CAD build for the part. Positions are in the model's coordinates, mm. A direction names the side the tool comes from. Round coordinates to 2 decimals unless told otherwise and drop trailing zeros. Order: outer loops, then holes, each group sorted by start corner. A loop starts at its lowest first (then second) coordinate and runs counter-clockwise, first axis right, second up. Notation, with made-up numbers: (39, -34) -> (92, -34) arc R21 cw to (92, -23) -> close; hole circle Ø8 at (-37, 1). An arc over 180 degrees is marked (long way). Return JSON: item names as keys, results as strings. Group by question number.
Q1. Which spindle directions (+Z, -Z, +X, -X, +Y, -Y) get a long thin tool onto all of the face, cutting with end or side? Do faces 4 (the flat face through (-27, 64, 5)), 5 (the flat face through (19, 240, -4)). Say none if no direction does.
Q2. Cut at B-B (x = 0). Write the cut outline in (y, z).
Q3. Cut at A-A (z = 0). Write the cut outline in (x, y).
Q4. Cut at D-D (x = 31). Count the separate pieces of the cut face and the enclosed holes in it, then the cut area to 3 significant figures.
Q5. Mould opens along Z. For faces 1 (the flat face through (27, 156, 0)), 2 (the cylindrical face through (-34.168, 118.46, -7.587)), 3 (the flat face through (19, 0, -4)) say: +Z half, -Z half, draft (parallel to the pull), parting line (faces both ways), or undercut.
Q6. Cut at C-C (y = 54). Write the cut outline in (x, z).
Q7. Probe line 1 along Y through (x, z) = (-29, 0.5); line 2 along Z through (x, y) = (-24.5, 75.5) (3 decimals); line 3 along Y through (x, z) = (4, 25.5). List the from-to ranges inside material, lowest first.
Q8. Flat gauge pins, fed straight in: pin 1 (8 mm diameter, centred on x = -29.5, z = 0.5, fed in from +Y); pin 2 (5 mm diameter, centred on x = -28.5, y = 180.5, fed in from +Z); pin 3 (3 mm diameter, centred on x = 8, y = 134, fed in from -Z). Where does each tip first touch, or does it go through?
from build123d import *

# Parameters (mm, degrees)
SKETCH3_R               = 35
SKETCH3_R_2             = 19
BOSS_EXTRUDE2_DEPTH     = 240
CUT_EXTRUDE2_DEPTH      = 246.051015097
CUT_EXTRUDE2_DEPTH_BACK = 246.051015097
SKETCH5_W               = 10
SKETCH5_H               = 40
CUT_EXTRUDE3_DEPTH      = 246.051015097
CUT_EXTRUDE3_DEPTH_BACK = 246.051015097
SKETCH6_W               = 10
SKETCH6_H               = 40
FILLET2_R               = 10
FILLET3_R               = 10


with BuildPart() as part:
    # Sketch3 → Boss-Extrude2 (new body)
    with BuildSketch(Plane(origin=(0, 0, 0), x_dir=(1, 0, 0), z_dir=(0, 1, 0))):
        with Locations(Location((0, 0, 0), (0, 0, 270))):
            Circle(SKETCH3_R)
        with Locations(Location((0, 0, 0), (0, 0, 270))):
            Circle(SKETCH3_R_2, mode=Mode.SUBTRACT)
    extrude(amount=BOSS_EXTRUDE2_DEPTH)

    # Sketch5 → Cut-Extrude2 (cut, two sides: drawn at the far end of the back side and taken through both)
    with BuildSketch(Plane(origin=(0, 0, 0), x_dir=(0, 0, -1), z_dir=(1, 0, 0)).offset(-CUT_EXTRUDE2_DEPTH_BACK)):
        with Locations((0, 176)):
            Rectangle(SKETCH5_W, SKETCH5_H)
    extrude(amount=CUT_EXTRUDE2_DEPTH + CUT_EXTRUDE2_DEPTH_BACK, mode=Mode.SUBTRACT)

    # Sketch6 → Cut-Extrude3 (cut, two sides: drawn at the far end of the back side and taken through both)
    with BuildSketch(Plane(origin=(0, 0, 0), x_dir=(0, 0, -1), z_dir=(1, 0, 0)).offset(-CUT_EXTRUDE3_DEPTH_BACK)):
        with Locations((0, 64)):
            Rectangle(SKETCH6_W, SKETCH6_H)
    extrude(amount=CUT_EXTRUDE3_DEPTH + CUT_EXTRUDE3_DEPTH_BACK, mode=Mode.SUBTRACT)

    # Fillet2
    fillet2_edges = [part.edges().sort_by_distance(p)[0] for p in [
        (0, 240, -35),
    ]]
    fillet(fillet2_edges, radius=FILLET2_R)

    # Fillet3
    fillet3_edges = [part.edges().sort_by_distance(p)[0] for p in [
        (0, 0, -35),
    ]]
    fillet(fillet3_edges, radius=FILLET3_R)


solid = part.part
Solution:
{
 "1": {"face 4": "+X, -X", "face 5": "+Z, -Z, +X, -X, +Y"},
 "2": {"outline": "(0, -25) arc R10 ccw to (10, -35) -> (230, -35) arc R10 ccw to (240, -25) -> (240, -19) -> (0, -19) -> close; (0, 19) -> (240, 19) -> (240, 25) arc R10 ccw to (230, 35) -> (10, 35) arc R10 ccw to (0, 25) -> close"},
 "3": {"outline": "(-35, 10) arc R10 ccw to (-25, 0) -> (-19, 0) -> (-19, 44) -> (-35, 44) -> close; (-35, 84) -> (-19, 84) -> (-19, 156) -> (-35, 156) -> close; (-35, 196) -> (-19, 196) -> (-19, 240) -> (-25, 240) arc R10 ccw to (-35, 230) -> close; (19, 0) -> (25, 0) arc R10 ccw to (35, 10) -> (35, 44) -> (19, 44) -> close; (19, 84) -> (35, 84) -> (35, 156) -> (19, 156) -> close; (19, 196) -> (35, 196) -> (35, 230) arc R10 ccw to (25, 240) -> (19, 240) -> close"},
 "4": {"separate pieces": "1", "enclosed holes": "2", "area": "6,770 mm²"},
 "5": {"face 1": "undercut", "face 2": "parting line", "face 3": "draft"},
 "6": {"outline": "(-34.64, -5) arc R35 ccw to (34.64, -5) -> (18.33, -5) arc R19 cw to (-18.33, -5) -> close; (-34.64, 5) -> (-18.33, 5) arc R19 cw to (18.33, 5) -> (34.64, 5) arc R35 ccw to start"},
 "7": {"line 1": "y = 0.84 to 44, 84 to 156, 196 to 239.16", "line 2": "z = -24.995 to -5, 5 to 24.995", "line 3": "y = 0.03 to 239.97"},
 "8": {"pin 1": "stops at y = 239.99", "pin 2": "stops at z = 23.43", "pin 3": "stops at z = -34.39"}
}
